```python
from build123d import *

# Parameters (mm, degrees)
SALIENTE_EXTRUIR1_DEPTH = 12.7
CROQUIS2_R              = 3
CORTAR_EXTRUIR1_DEPTH   = 3
CROQUIS3_R              = 10
CROQUIS3_R_2            = 2
CORTAR_EXTRUIR2_DEPTH   = 31
CROQUIS4_R              = 1.5
CORTAR_EXTRUIR3_DEPTH   = 31
CROQUIS5_R              = 4
CORTAR_EXTRUIR4_DEPTH   = 3


with BuildPart() as part:
    # Croquis1 → Saliente-Extruir1 (new body)
    with BuildSketch(Plane.XY):
        with BuildLine():
            Line((10, 0), (90, 0))
            ThreePointArc((90, 0), (97.071067812, 2.928932188), (100, 10))
            Line((100, 10), (100, 90))
            ThreePointArc((100, 90), (97.071067812, 97.071067812), (90, 100))
            Line((90, 100), (10, 100))
            ThreePointArc((10, 100), (2.928932188, 97.071067812), (0, 90))
            Line((0, 90), (0, 10))
            ThreePointArc((0, 10), (2.928932188, 2.928932188), (10, 0))
        make_face()
    extrude(amount=SALIENTE_EXTRUIR1_DEPTH)

    # Croquis2 → Cortar-Extruir1 (cut)
    with BuildSketch(Plane.XY.offset(12.7)):
        with Locations((10, 90)):
            Circle(CROQUIS2_R)
        with Locations((10, 10)):
            Circle(CROQUIS2_R)
        with Locations((90, 90)):
            Circle(CROQUIS2_R)
        with Locations((90, 10)):
            Circle(CROQUIS2_R)
    extrude(amount=-CORTAR_EXTRUIR1_DEPTH, mode=Mode.SUBTRACT)

    # Croquis3 → Cortar-Extruir2 (cut)
    with BuildSketch(Plane.XY.offset(12.7)):
        with Locations((50, 50)):
            Circle(CROQUIS3_R)
        with Locations((26.43, 73.57)):
            Circle(CROQUIS3_R_2)
        with Locations((73.57, 73.57)):
            Circle(CROQUIS3_R_2)
        with Locations((26.43, 26.43)):
            Circle(CROQUIS3_R_2)
        with Locations((73.57, 26.43)):
            Circle(CROQUIS3_R_2)
    extrude(amount=-CORTAR_EXTRUIR2_DEPTH, mode=Mode.SUBTRACT)

    # Croquis4 → Cortar-Extruir3 (cut)
    with BuildSketch(Plane.XY.offset(9.7)):
        with Locations((10, 90)):
            Circle(CROQUIS4_R)
        with Locations((90, 90)):
            Circle(CROQUIS4_R)
        with Locations((90, 10)):
            Circle(CROQUIS4_R)
        with Locations((10, 10)):
            Circle(CROQUIS4_R)
    extrude(amount=-CORTAR_EXTRUIR3_DEPTH, mode=Mode.SUBTRACT)

    # Croquis5 → Cortar-Extruir4 (cut)
    with BuildSketch(Plane(origin=(0, 0, 0), x_dir=(-1, 0, 0), z_dir=(0, 0, -1))):
        with Locations((-73.57, 73.57)):
            Circle(CROQUIS5_R)
        with Locations((-26.43, 73.57)):
            Circle(CROQUIS5_R)
        with Locations((-26.43, 26.43)):
            Circle(CROQUIS5_R)
        with Locations((-73.57, 26.43)):
            Circle(CROQUIS5_R)
    extrude(amount=-CORTAR_EXTRUIR4_DEPTH, mode=Mode.SUBTRACT)


solid = part.part
```
For this review, take the finished solid that the model builds, in its own axes (mm). A direction names the side the tool comes from. Give positions to 0.01 mm unless a question says otherwise; leave off trailing zeros. Write each loop counter-clockwise with the first axis right and the second up, starting at its lowest first coordinate (ties: lowest second). Pieces come first, ordered by that corner, then holes. Notation, with made-up numbers: M -37.75,-1 L -14.75,-1 A17 ccw -14.75,22 Z; hole C 14.25,85 d4. An arc over 180 degrees is marked long. Answer as a JSON object with one key per item and string values. Group by question number.
Item 1: Consider section D-D on y = 50. Write out the cut boundary in (x, z).
Item 2: Draft analysis for pull direction X (two halves, no side actions). For faces 1 (the flat face through (51, 100, 6)), 2 (the cylindrical face through (22.615, 27.631, 1.479)), 3 (the cylindrical face through (87.6, 88.2, 11.2)), 4 (the flat face through (0, 51, 6)), state which applies: +X half, -X half, draft (parallel to the pull), parting line (faces both ways), or undercut.
Item 3: For pin 1 Ø4.5 at (x, y) = (26.43, 26.43) entering from -Z; pin 2 Ø2.5 at (x, y) = (74, 74) entering from -Z, all flat-tipped, find the tip position at first contact; note any pin that passes through.
Item 4: Consider section A-A on z = 6.75. Count the separate pieces of the cut face and the enclosed holes in it, plus the area to 3 significant figures.
Item 5: For probe 1 along Y at (x, z) = (73.57, 1.5); probe 2 along Y at (x, z) = (10, 6), list the stretches that pass through material, from the lowest coordinate up. Write a range as [from, to].
Item 6: Consider section B-B on y = 26.43. Write out the cut boundary in (x, z), plus the area to 3 significant figures.
Item 7: Tool access review of faces 5 (the cylindrical face through (76.52, 29.13, 1.48)), 6 (the cylindrical face through (9.805, 91.487, 4.918)), 7 (the cylindrical face through (9.35, 87.07, 11.22)): name each direction out of +Z, -Z, +X, -X, +Y, -Y from which nothing blocks a thin tool from reaching the whole face with its end or side.
Check result:
{
 "1": {"outline": "M 0,0 L 40,0 L 40,12.7 L 0,12.7 Z; M 60,0 L 100,0 L 100,12.7 L 60,12.7 Z"},
 "2": {"face 1": "draft", "face 2": "undercut", "face 3": "undercut", "face 4": "-X half"},
 "3": {"pin 1": "stops at z = 3", "pin 2": "passes through"},
 "4": {"separate pieces": "1", "enclosed holes": "9", "area": "9,520 mm^2"},
 "5": {"probe 1": "y = [0, 22.43], [30.43, 69.57], [77.57, 100]", "probe 2": "y = [0, 8.5], [11.5, 88.5], [91.5, 100]"},
 "6": {"outline": "M 0,0 L 22.43,0 L 22.43,3 L 24.43,3 L 24.43,12.7 L 0,12.7 Z; M 28.43,3 L 30.43,3 L 30.43,0 L 69.57,0 L 69.57,3 L 71.57,3 L 71.57,12.7 L 28.43,12.7 Z; M 75.57,3 L 77.57,3 L 77.57,0 L 100,0 L 100,12.7 L 75.57,12.7 Z", "area": "1,140 mm^2"},
 "7": {"face 5": "-Z", "face 6": "+Z, -Z", "face 7": "+Z"}
}
